from build123d import *

# Parameters (mm, degrees)
SKETCH1_R          = 3.5
SKETCH1_R_2        = 1.5
SKETCH1_R_3        = 1.75
BASE_FLANGE1_DEPTH = 5
FILLET1_R          = 10


# Sheet-metal steps are written as plain solids
with BuildPart() as part:
    # Sketch1 → Base-Flange1 (new body)
    with BuildSketch(Plane.XY):
        with BuildLine():
            Line((7.071067812, 2.5), (39.287857357, 2.5))
            ThreePointArc((39.287857357, 2.5), (61, 0), (39.287857357, -2.5))
            Line((39.287857357, -2.5), (7.071067812, -2.5))
            ThreePointArc((7.071067812, -2.5), (-7.5, 0), (7.071067812, 2.5))
        make_face()
        Circle(SKETCH1_R, mode=Mode.SUBTRACT)
        with Locations((50, 8)):
            Circle(SKETCH1_R_2, mode=Mode.SUBTRACT)
        with Locations((58, 0)):
            Circle(SKETCH1_R_2, mode=Mode.SUBTRACT)
        with Locations((50, -8)):
            Circle(SKETCH1_R_2, mode=Mode.SUBTRACT)
        with Locations((42, 0)):
            Circle(SKETCH1_R_2, mode=Mode.SUBTRACT)
        with Locations((50, 0)):
            Circle(SKETCH1_R_3, mode=Mode.SUBTRACT)
    extrude(amount=-BASE_FLANGE1_DEPTH)

    # Fillet1
    fillet1_edges = [part.edges().sort_by_distance(p)[0] for p in [
        (7.071067812, 2.5, -2.5),
        (39.287857357, 2.5, -2.5),
        (39.287857357, -2.5, -2.5),
        (7.071067812, -2.5, -2.5),
    ]]
    fillet(fillet1_edges, radius=FILLET1_R)


solid = part.part
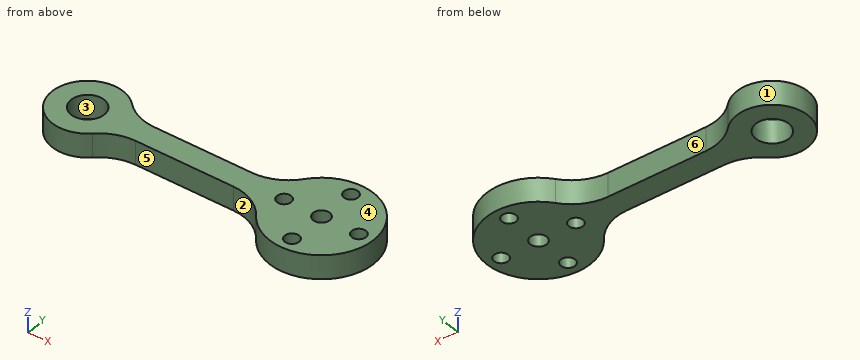
For this review, take the finished solid that the model builds, in its own axes (mm). Face numbers are marked on the shaded views. A direction names the side the tool comes from. Round coordinates to 2 decimals unless told otherwise and drop trailing zeros. Loops run counter-clockwise (first coordinate to the right, second up) from the corner with the lowest first, then second, coordinate; pieces in that order, holes last. Notation, with made-up numbers: (-4.5, 1.25) - (4.5, 1.25) arc R20 cw to (4.5, 36.25) - close; hole circle Ø6 at (-9.75, -25.75). An arc over 180 degrees is marked (long way). One line per item, written item: value. Start each with the question number.
Item 1: Take a section at D-D (y = 8.75). Give the boundary of the cut face in (x, z).
Item 2: For L1, parallel to Y at x = 50, z = -1.85; L2, parallel to X at y = -4.5, z = -4.05; L3, parallel to X at y = -8.5, z = -4, list the stretches that pass through material, from the lowest coordinate up.
Item 3: Take a section at C-C (z = -3.5). Give the boundary of the cut face in (x, y), plus the area to 3 significant figures.
Item 4: Take a section at B-B (y = 0). Give the boundary of the cut face in (x, z).
Item 5: Take a section at A-A (x = 0). Give the boundary of the cut face in (y, z).
Item 6: The part is to be moulded in two halves that separate along Y. For the marked faces 1, 2 and 3, say which applies: +Y half, -Y half, draft (parallel to the pull), parting line (faces both ways), or undercut.
Item 7: For the marked faces 4, 5 and 6, list the 3-axis set-ups (+Z, -Z, +X, -X, +Y, -Y) from which the entire face can be reached by the end or side of a thin tool; tool diameter is ignored.
Item 8: Clearance check with flat-ended pins moving along their axes: pin 1 Ø2.5 at (x, y) = (50, 8) entering from -Z; pin 2 Ø2 at (y, z) = (-7.5, -2) entering from -X; pin 3 Ø1 at (y, z) = (-5, -2) entering from -X. State where each tip first meets the part, or that it passes through.
Answer below:
1. outline: (43.33, -5) - (48.7, -5) - (48.7, 0) - (43.33, 0) - close; (51.3, -5) - (56.67, -5) - (56.67, 0) - (51.3, 0) - close
2. L1: y = -11 to -9.5, -6.5 to -1.75, 1.75 to 6.5, 9.5 to 11
2. L2: x = -6 to 6.25, 39.13 to 60.04
2. L3: x = 43.02 to 48.59, 51.41 to 56.98
3. outline: (5.25, -5.36) arc R10 cw to (12.25, -2.5) - (33.13, -2.5) arc R10 cw to (41.16, -6.55) arc R11 ccw (long way) to (41.16, 6.55) arc R10 cw to (33.13, 2.5) - (12.25, 2.5) arc R10 cw to (5.25, 5.36) arc R7.5 ccw (long way) to start; hole circle Ø7 at (0, 0); hole circle Ø3 at (42, 0); hole circle Ø3.5 at (50, 0); hole circle Ø3 at (50, -8); hole circle Ø3 at (50, 8); hole circle Ø3 at (58, 0)
3. area: 656 mm2
4. outline: (-7.5, -5) - (-3.5, -5) - (-3.5, 0) - (-7.5, 0) - close; (3.5, -5) - (40.5, -5) - (40.5, 0) - (3.5, 0) - close; (43.5, -5) - (48.25, -5) - (48.25, 0) - (43.5, 0) - close; (51.75, -5) - (56.5, -5) - (56.5, 0) - (51.75, 0) - close; (59.5, -5) - (61, -5) - (61, 0) - (59.5, 0) - close
5. outline: (-7.5, -5) - (-3.5, -5) - (-3.5, 0) - (-7.5, 0) - close; (3.5, -5) - (7.5, -5) - (7.5, 0) - (3.5, 0) - close
6. face 1: parting line
6. face 2: -Y half
6. face 3: undercut
7. face 4: +Z, +X, -X, +Y, -Y
7. face 5: +Z, -Z, -Y
7. face 6: +Z, -Z, +Y
8. pin 1: passes through
8. pin 2: stops at x = -3.74
8. pin 3: stops at x = -6
